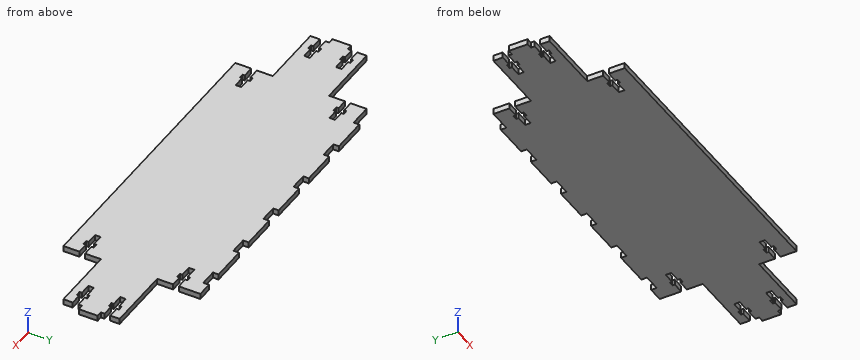
from build123d import *

# Parameters (mm, degrees)
SKETCH_1_W             = 160
SKETCH_1_H             = 70
EXTRUDE_1_DEPTH        = 3
EXTRUDE_2_DEPTH        = 35
EXTRUDE_2_DEPTH_BACK   = 195
SKETCH_2_W             = 3
SKETCH_2_H             = 30
EXTRUDE_3_DEPTH        = 3
EXTRUDE_3_DEPTH_BACK   = 233
SKETCH_3_W             = 3
SKETCH_3_H             = 10
CUT_EXTRUDE_1_DEPTH    = 3
CUT_EXTRUDE_2_DEPTH    = 3
SKETCH_6_W             = 8
SKETCH_6_H             = 3
EXTRUDE_4_DEPTH        = 3
SKETCH_7_W             = 19
SKETCH_7_H             = 3
EXTRUDE_5_DEPTH        = 3
PATTERN_LINEAR_1_COUNT = 5
PATTERN_LINEAR_1_PITCH = 28


with BuildPart() as part:
    # Эскиз1 → Бобышка-Вытянуть1 (new body)
    with BuildSketch(Plane.XY):
        with Locations((80, 35)):
            Rectangle(SKETCH_1_W, SKETCH_1_H)
    extrude(amount=EXTRUDE_1_DEPTH)

    # Эскиз2 → Бобышка-Вытянуть2 (add, two sides: drawn at the far end of the back side and taken through both)
    with BuildSketch(Plane(origin=(160, 0, 0), x_dir=(0, 0, -1), z_dir=(1, 0, 0)).offset(-EXTRUDE_2_DEPTH_BACK)):
        with Locations((-1.5, 35)):
            Rectangle(SKETCH_2_W, SKETCH_2_H)
    extrude(amount=EXTRUDE_2_DEPTH + EXTRUDE_2_DEPTH_BACK)

    # Эскиз3 → Бобышка-Вытянуть3 (add, two sides: drawn at the far end of the back side and taken through both)
    with BuildSketch(Plane(origin=(195, 0, 0), x_dir=(0, 0, -1), z_dir=(1, 0, 0)).offset(-EXTRUDE_3_DEPTH_BACK)):
        with Locations((-1.5, 35)):
            Rectangle(SKETCH_3_W, SKETCH_3_H)
    extrude(amount=EXTRUDE_3_DEPTH + EXTRUDE_3_DEPTH_BACK)

    # Эскиз4 → Вырез-Вытянуть1 (cut)
    with BuildSketch(Plane.XY.offset(3)):
        Polygon((160, 58.5), (154, 58.5), (154, 57.25), (151.5, 57.25), (151.5, 58.5), (145.5, 58.5), (145.5, 61.5), (151.5, 61.5), (151.5, 62.75), (154, 62.75), (154, 61.5), (160, 61.5), align=None)
        Polygon((160, 8.5), (160, 11.5), (154, 11.5), (154, 12.75), (151.5, 12.75), (151.5, 11.5), (145.5, 11.5), (145.5, 8.5), (151.5, 8.5), (151.5, 7.25), (154, 7.25), (154, 8.5), align=None)
        Polygon((0, 11.5), (6, 11.5), (6, 12.75), (8.5, 12.75), (8.5, 11.5), (14.5, 11.5), (14.5, 8.5), (8.5, 8.5), (8.5, 7.25), (6, 7.25), (6, 8.5), (0, 8.5), align=None)
        Polygon((0, 61.5), (0, 58.5), (6, 58.5), (6, 57.25), (8.5, 57.25), (8.5, 58.5), (14.5, 58.5), (14.5, 61.5), (8.5, 61.5), (8.5, 62.75), (6, 62.75), (6, 61.5), align=None)
    extrude(amount=-CUT_EXTRUDE_1_DEPTH, mode=Mode.SUBTRACT)

    # Эскиз5 → Вырез-Вытянуть2 (cut)
    with BuildSketch(Plane.XY.offset(3)):
        Polygon((195, 45), (189, 45), (189, 46.25), (186.5, 46.25), (186.5, 45), (180.5, 45), (180.5, 42), (186.5, 42), (186.5, 40.75), (189, 40.75), (189, 42), (195, 42), align=None)
        Polygon((195, 28), (195, 25), (189, 25), (189, 23.75), (186.5, 23.75), (186.5, 25), (180.5, 25), (180.5, 28), (186.5, 28), (186.5, 29.25), (189, 29.25), (189, 28), align=None)
        Polygon((-35, 25), (-29, 25), (-29, 23.75), (-26.5, 23.75), (-26.5, 25), (-20.5, 25), (-20.5, 28), (-26.5, 28), (-26.5, 29.25), (-29, 29.25), (-29, 28), (-35, 28), align=None)
        Polygon((-35, 42), (-35, 45), (-29, 45), (-29, 46.25), (-26.5, 46.25), (-26.5, 45), (-20.5, 45), (-20.5, 42), (-26.5, 42), (-26.5, 40.75), (-29, 40.75), (-29, 42), align=None)
    extrude(amount=-CUT_EXTRUDE_2_DEPTH, mode=Mode.SUBTRACT)

    # Эскиз6 → Бобышка-Вытянуть4 (add)
    with BuildSketch(Plane(origin=(0, 70, 0), x_dir=(1, 0, 0), z_dir=(0, 1, 0))):
        with Locations((156, -1.5)):
            Rectangle(SKETCH_6_W, SKETCH_6_H)
    extrude(amount=EXTRUDE_4_DEPTH)

    # Эскиз7 → Бобышка-Вытянуть5 (add)
    with BuildSketch(Plane(origin=(0, 70, 0), x_dir=(1, 0, 0), z_dir=(0, 1, 0))):
        with Locations((133.5, -1.5)):
            Rectangle(SKETCH_7_W, SKETCH_7_H)
    extrude_5 = extrude(amount=EXTRUDE_5_DEPTH)

    # Линейный массив1: Бобышка-Вытянуть5 ×5
    with Locations(*[(-i * PATTERN_LINEAR_1_PITCH, 0, 0) for i in range(1, PATTERN_LINEAR_1_COUNT)]):
        add(extrude_5)


solid = part.part
For this review, take the finished solid that the model builds, in its own axes (mm). Give positions to 0.01 mm unless a question says otherwise; leave off trailing zeros. Order: outer loops, then holes, each group sorted by start corner. A loop starts at its lowest first (then second) coordinate and runs counter-clockwise, first axis right, second up. Notation, with made-up numbers: (51.5, 12.25) -> (61.5, 12.25) arc R27 ccw to (61.5, 30.25) -> close; hole circle Ø1 at (-39.5, 32). An arc over 180 degrees is marked (long way). Write item = value, one per line.
1) We need section A-A, the plane x = 177.5. Give the boundary of the cut face in (y, z).
Findings:
outline = (20, 0) -> (50, 0) -> (50, 3) -> (20, 3) -> close
2) Insertion check: pin 1 (0.9 mm diameter, centred on y = 14, z = 2, fed in from -X); pin 2 (1.4 mm diameter, centred on y = 28.5, z = 1, fed in from +X); pin 3 (0.9 mm diameter, centred on y = 26.5, z = 1, fed in from -X). Each pin has a flat end and moves straight along its axis. Give the tip position at first contact, or say it passes through.
Findings:
pin_1 = 0
pin_2 = 195
pin_3 = -20.5
3) We need section B-B, the plane y = 52.5. Give the boundary of the cut face in (x, z).
Findings:
outline = (0, 0) -> (160, 0) -> (160, 3) -> (0, 3) -> close
4) To check wall thickness, follow L1, parallel to X at y = 70.5, z = 0.1; L2, parallel to Y at x = 183.5, z = 0.3; L3, parallel to X at y = 57.5, z = 0.5. State the ranges of each line that lie inside material, in increasing order. Write a range as from..to.
Findings:
L1 = 12..31, 40..59, 68..87, 96..115, 124..143, 152..160
L2 = 20..25, 28..42, 45..50
L3 = 0..6, 8.5..151.5, 154..160
